```python
from build123d import *

# Parameters (mm, degrees)
EXTRUDE_1_DEPTH      = 1.95
EXTRUDE_1_DEPTH_BACK = 1.95
SKETCH_1_W           = 4.8
SKETCH_1_H           = 5.1
SKETCH_4_R           = 0.55
CUT_EXTRUDE_1_DEPTH  = 0.56
SKETCH_5_W           = 1.288637745
SKETCH_5_H           = 1.3
SKETCH_5_W_2         = 1.014010029
SKETCH_5_H_2         = 0.602068455
EXTRUDE_1_2_DEPTH    = 0.2


with BuildPart() as part:
    # 草图1 → Extrude 1 (new, two sides: drawn at the far end of the back side and taken through both)
    with BuildSketch(Plane(origin=(0, 0, 0), x_dir=(1, 0, 0), z_dir=(0, 1, 0)).offset(-EXTRUDE_1_DEPTH_BACK)):
        Rectangle(SKETCH_1_W, SKETCH_1_H)
    extrude(amount=EXTRUDE_1_DEPTH + EXTRUDE_1_DEPTH_BACK)

    # 草图4 → 切除-拉伸1 (cut)
    with BuildSketch(Plane.XY.offset(2.55)):
        with Locations((-1.52, 0.65)):
            Circle(SKETCH_4_R)
    extrude(amount=-CUT_EXTRUDE_1_DEPTH, mode=Mode.SUBTRACT)

    # 草图5 → Extrude 1 2 (add)
    with BuildSketch(Plane(origin=(0, 0, -2.55), x_dir=(-1, 0, 0), z_dir=(0, 0, -1))):
        with Locations((-1.922058583, 0)):
            Rectangle(SKETCH_5_W, SKETCH_5_H)
        with Locations((2.092994985, 1.359060107)):
            Rectangle(SKETCH_5_W_2, SKETCH_5_H_2)
        with Locations((2.092994985, -1.359060107)):
            Rectangle(SKETCH_5_W_2, SKETCH_5_H_2)
    extrude(amount=EXTRUDE_1_2_DEPTH)


solid = part.part
```
Geometry: final body of the model. Coordinates: model frame, mm. A direction names the side the tool comes from. Coordinates: 2 decimals unless noted, no trailing zeros. Loops run counter-clockwise (first coordinate to the right, second up) from the corner with the lowest first, then second, coordinate; pieces in that order, holes last. Notation, with made-up numbers: (65.25, -12) -> (118.25, -12) arc R15 cw to (118.25, 15) -> close; hole circle Ø7 at (-35.75, 55). An arc over 180 degrees is marked (long way). Use a Markdown table: item, result. Add a question column.
(1) Section query D-D, the plane x = -1.95. Return loops of the section in (y, z), plus the area to 3 significant figures.
(2) Pin query (flat end, axial travel): pin 1 Ø1.2 at (y, z) = (0.5, -0.5) entering from -X; pin 2 Ø1 at (x, y) = (-0.5, 0.5) entering from -Z; pin 3 Ø1.2 at (y, z) = (1, -1) entering from +X. Return the tip coordinate at first contact, or that it passes through.
(3) Section query A-A, the plane x = 1.9. Return loops of the section in (y, z).
(4) Mould query, pull axis Y, two halves, no side actions, for faces 5 (the flat face through (2, 0, -2.75)), 6 (the flat face through (0, 0, -2.55)), 7 (the flat face through (0, 1.95, 0)), 8 (the cylindrical face through (-1.925, 1.022, 2.274)). Classes: pulls with the +Y half, pulls with the -Y half, needs draft (parallel to the pull), parting line crosses it, or undercut.
(5) Line query: line 1 along Y through (x, z) = (-1.52, 2.25); line 2 along X through (y, z) = (-1.5, 1.6); line 3 along Z through (x, y) = (0.95, -1.15). Output: solid intervals per line, ascending.
(6) Access query for faces 1 (the flat face through (-2.4, 0, 0)), 2 (the flat face through (0, -1.95, 0)), 3 (the flat face through (2.4, 0, 0)), 4 (the flat face through (-1.5, 0.7, 1.99)). Directions: +Z, -Z, +X, -X, +Y, -Y. A direction counts if a zero-diameter tool reaches every point of the face in a straight line with its end or side. Return the directions, or none.
(7) Section query B-B, the plane z = 2.1. Return loops of the section in (x, y).
(8) Section query C-C, the plane y = -0.5. Return loops of the section in (x, z), plus the area to 3 significant figures.
Answer:
| question | item | result |
|---|---|---|
| 1 | outline | (-1.95, -2.55) -> (-1.66, -2.55) -> (-1.66, -2.75) -> (-1.06, -2.75) -> (-1.06, -2.55) -> (1.06, -2.55) -> (1.06, -2.75) -> (1.66, -2.75) -> (1.66, -2.55) -> (1.95, -2.55) -> (1.95, 2.55) -> (0.99, 2.55) -> (0.99, 1.99) -> (0.31, 1.99) -> (0.31, 2.55) -> (-1.95, 2.55) -> close |
| 1 | area | 19.7 mm^2 |
| 2 | pin 1 | stops at x = -2.4 |
| 2 | pin 2 | stops at z = -2.55 |
| 2 | pin 3 | stops at x = 2.4 |
| 3 | outline | (-1.95, -2.55) -> (-0.65, -2.55) -> (-0.65, -2.75) -> (0.65, -2.75) -> (0.65, -2.55) -> (1.95, -2.55) -> (1.95, 2.55) -> (-1.95, 2.55) -> close |
| 4 | face 5 | needs draft |
| 4 | face 6 | undercut |
| 4 | face 7 | pulls with the +Y half |
| 4 | face 8 | undercut |
| 5 | line 1 | y = -1.95 to 0.1, 1.2 to 1.95 |
| 5 | line 2 | x = -2.4 to 2.4 |
| 5 | line 3 | z = -2.55 to 2.55 |
| 6 | face 1 | +Z, -X, +Y, -Y |
| 6 | face 2 | +Z, -Z, +X, -X, -Y |
| 6 | face 3 | +Z, +X, +Y, -Y |
| 6 | face 4 | +Z |
| 7 | outline | (-2.4, -1.95) -> (2.4, -1.95) -> (2.4, 1.95) -> (-2.4, 1.95) -> close; hole circle Ø1.1 at (-1.52, 0.65) |
| 8 | outline | (-2.4, -2.55) -> (1.28, -2.55) -> (1.28, -2.75) -> (2.57, -2.75) -> (2.57, -2.55) -> (2.4, -2.55) -> (2.4, 2.55) -> (-2.4, 2.55) -> close |
| 8 | area | 24.7 mm^2 |
